Autodesk Inventor part; units mm, degrees
ref_plane "YZ Plane" through (0, 0, 0) normal (1, 0, 0) x (0, 1, 0)
ref_plane "XZ Plane" through (0, 0, 0) normal (0, 1, 0) x (-1, 0, 0)
ref_plane "XY Plane" through (0, 0, 0) normal (0, 0, 1) x (1, 0, 0)
sketch "Sketch1" plane through (0, 0, 0) normal (0, 0, 1) x (1, 0, 0)
  circle A0 centre (0, 0) radius 7.9375
  circle A1 centre (0, 0) radius 3.175
extrude "Extrusion1" add sketch "Sketch1" along normal blind 6.35
sketch "Sketch2" plane through (0, 0, 6.35) normal (0, 0, 1) x (1, 0, 0)
  circle A0 centre (0, 0) radius 3.175
  circle A1 centre (0, 0) radius 7.9375
  circle A2 centre (0, 0) radius 11.1125
extrude "Extrusion2" add sketch "Sketch2" along normal blind 6.35 contours A1 | A2
sketch "Sketch3" plane through (0, 0, 12.7) normal (0, 0, 1) x (1, 0, 0)
  circle A0 centre (0, 0) radius 3.175
  circle A1 centre (0, 0) radius 11.1125
  circle A2 centre (0, 0) radius 9.525
extrude "Extrusion3" add sketch "Sketch3" along normal blind 3.175 contours A2
chamfer "Chamfer1" distance 0.254 angle 45 6 edges at (-9.525, 0, 15.875) (-3.175, 0, 15.875) (-11.1125, 0, 12.7) (-11.1125, 0, 6.35) (-7.9375, 0, 0) (-3.175, 0, 0)
properties part number "cyl head"
Model file for the job. Use its own axes, mm. A direction names the side the tool comes from. Give positions to 0.01 mm unless a question says otherwise; leave off trailing zeros. Order: outer loops, then holes, each group sorted by start corner. A loop starts at its lowest first (then second) coordinate and runs counter-clockwise, first axis right, second up. Notation, with made-up numbers: M 70,72 L 116,72 A27 cw 116,108 Z; hole C 15.5,-12.75 d9. An arc over 180 degrees is marked long. Put each result on its own line as item: value. Start each with the question number.
(1) Tool access for faces 1 (the face through (-2, -8, 6.35)), 2 (the face through (10.6, -3.34, 9.48)): list every direction of +Z, -Z, +X, -X, +Y, -Y with a clear straight run to the whole face (end or side of a thin tool).
(2) Pull direction Y, two halves, no side cores. Call faces 3 (the face through (-7.559, 5.796, 14.14)), 4 (the face through (-0.69, 3.1, 7.83)), 5 (the face through (0, -10, 12.7)): released by +Y, released by -Y, zero draft, split by the parting line, or undercut.
(3) Pin check, flat tips, straight feed: pin 1 Ø1 at (x, z) = (-2.5, 3) entering from +Y; pin 2 Ø5 at (x, z) = (3, 6.5) entering from +Y; pin 3 Ø6 at (y, z) = (-8, 2.5) entering from -X; pin 4 Ø6.5 at (x, y) = (2.5, -2) entering from +Z (3 decimals). Stop position of each tip, or through.
(4) Band-saw the part on C-C on z = 13.25. Give the cut face in (x, y) (3 decimals), then the cut area to 3 significant figures.
(5) Drill centre lines: L1, parallel to Y at x = 0, z = 4.25 (1 decimal); L2, parallel to Y at x = 0, z = 9.25 (1 decimal); L3, parallel to Z at x = 8.25, y = -6.75. Where is each one in solid material? Low to high. Write a range as [from, to].
Results below:
1. face 1: -Z
1. face 2: +Z, -Z
2. face 3: split by the parting line
2. face 4: undercut
2. face 5: zero draft
3. pin 1: stops at y = 7.68
3. pin 2: stops at y = 11.1
3. pin 3: stops at x = -6.16
3. pin 4: stops at z = 15.875
4. outline: C 0,0 d19.05; hole C 0,0 d6.35
4. area: 253 mm2
5. L1: y = [-7.9, -3.2], [3.2, 7.9]
5. L2: y = [-11.1, -3.2], [3.2, 11.1]
5. L3: z = [6.35, 12.7]
